Autodesk Inventor part; units mm, degrees
ref_plane "YZ Plane" through (0, 0, 0) normal (1, 0, 0) x (0, 1, 0)
ref_plane "XZ Plane" through (0, 0, 0) normal (0, 1, 0) x (-1, 0, 0)
ref_plane "XY Plane" through (0, 0, 0) normal (0, 0, 1) x (1, 0, 0)
sketch "Boceto1" plane through (0, 0, 0) normal (0, 1, 0) x (-1, 0, 0)
  circle A0 centre (-59.7419, -103.4763) radius 7.9656
  circle A1 centre (-47.2958, -81.9187) radius 1.9914
  line L0 (-73.6817, -103.4763) -> (-73.6817, 5.1739)
  line L1 (32.3603, -66.3972) -> (-52.772, -115.5485)
  arc A2 (-73.6817, -103.4763) -> (-52.772, -115.5485) centre (-59.7419, -103.4763) ccw
  line L2 (13.9398, -24.1443) -> (18.9183, -32.7673)
  line L3 (20.9097, -36.2166) -> (25.8882, -44.8396)
  line L4 (27.8796, -48.2888) -> (32.8581, -56.9118)
  line L5 (7.5794, -22.7716) -> (11.1559, -28.9662)
  line L6 (11.1559, -28.9662) -> (13.9398, -24.1443)
  line L7 (13.9398, -24.1443) -> (18.9183, -32.7673)
  line L8 (18.9183, -32.7673) -> (12.9441, -32.7673)
  line L9 (12.9441, -32.7673) -> (17.9226, -41.3904)
  line L10 (17.9226, -41.3904) -> (20.9097, -36.2166)
  line L11 (20.9097, -36.2166) -> (25.8882, -44.8396)
  line L12 (25.8882, -44.8396) -> (19.914, -44.8396)
  line L13 (19.914, -44.8396) -> (24.8925, -53.4626)
  line L14 (24.8925, -53.4626) -> (27.8796, -48.2888)
  line L15 (27.8796, -48.2888) -> (32.8581, -56.9118)
  line L16 (32.8581, -56.9118) -> (26.8839, -56.9118)
  line L17 (26.8839, -56.9118) -> (32.3603, -66.3972)
  line L18 (-27.8795, 0.0001) -> (-37.8365, 0.0001)
  line L19 (-41.8193, 0.0001) -> (-51.7763, 0.0001)
  line L20 (-55.7591, 0.0001) -> (-65.7161, 0.0001)
  line L21 (-23.4355, 5.1739) -> (-30.8666, 5.1739)
  line L22 (-30.8666, 5.1739) -> (-27.8795, 0.0001)
  line L23 (-27.8795, 0.0001) -> (-37.8365, 0.0001)
  line L24 (-37.8365, 0.0001) -> (-34.8494, 5.1739)
  line L25 (-34.8494, 5.1739) -> (-44.8064, 5.1739)
  line L26 (-44.8064, 5.1739) -> (-41.8193, 0.0001)
  line L27 (-41.8193, 0.0001) -> (-51.7763, 0.0001)
  line L28 (-51.7763, 0.0001) -> (-48.7892, 5.1739)
  line L29 (-48.7892, 5.1739) -> (-58.7462, 5.1739)
  line L30 (-58.7462, 5.1739) -> (-55.7591, 0.0001)
  line L31 (-55.7591, 0.0001) -> (-65.7161, 0.0001)
  line L32 (-65.7161, 0.0001) -> (-62.729, 5.1739)
  line L33 (-62.729, 5.1739) -> (-73.6817, 5.1739)
  arc A3 (-23.4355, 5.1739) -> (7.5794, -22.7716) centre (0, 0) ccw
extrude "Extrusión2" add sketch "Boceto1" along normal blind 10
sketch "Boceto2" plane through (0, 10, 0) normal (0, 1, 0) x (1, 0, 0)
  circle A0 centre (59.7419, 103.4763) radius 7.9656
  circle A1 centre (47.2958, 81.9187) radius 1.9914
  arc A2 (73.6817, 103.4763) -> (52.772, 115.5485) centre (59.7419, 103.4763) ccw
  line L0 (52.772, 115.5485) -> (-32.3603, 66.3972)
  line L1 (-32.3603, 66.3972) -> (-26.8839, 56.9118)
  line L2 (-26.8839, 56.9118) -> (-32.8581, 56.9118)
  line L3 (-32.8581, 56.9118) -> (-27.8796, 48.2888)
  line L4 (-27.8796, 48.2888) -> (-24.8925, 53.4626)
  line L5 (-24.8925, 53.4626) -> (-19.914, 44.8396)
  line L6 (-19.914, 44.8396) -> (-25.8882, 44.8396)
  line L7 (-25.8882, 44.8396) -> (-20.9097, 36.2166)
  line L8 (-20.9097, 36.2166) -> (-17.9226, 41.3904)
  line L9 (-17.9226, 41.3904) -> (-12.9441, 32.7673)
  line L10 (-12.9441, 32.7673) -> (-18.9183, 32.7673)
  line L11 (-18.9183, 32.7673) -> (-13.9398, 24.1443)
  line L12 (-13.9398, 24.1443) -> (-11.1559, 28.9662)
  line L13 (-11.1559, 28.9662) -> (-7.5794, 22.7716)
  arc A3 (23.4355, -5.1739) -> (-7.5794, 22.7716) centre (0, 0) ccw
  line L14 (23.4355, -5.1739) -> (30.8666, -5.1739)
  line L15 (30.8666, -5.1739) -> (27.8795, -0.0001)
  line L16 (27.8795, -0.0001) -> (37.8365, -0.0001)
  line L17 (37.8365, -0.0001) -> (34.8494, -5.1739)
  line L18 (34.8494, -5.1739) -> (44.8064, -5.1739)
  line L19 (44.8064, -5.1739) -> (41.8193, -0.0001)
  line L20 (41.8193, -0.0001) -> (51.7763, -0.0001)
  line L21 (51.7763, -0.0001) -> (48.7892, -5.1739)
  line L22 (48.7892, -5.1739) -> (58.7462, -5.1739)
  line L23 (58.7462, -5.1739) -> (55.7591, -0.0001)
  line L24 (55.7591, -0.0001) -> (65.7161, -0.0001)
  line L25 (65.7161, -0.0001) -> (62.729, -5.1739)
  line L26 (62.729, -5.1739) -> (73.6817, -5.1739)
  line L27 (73.6817, -5.1739) -> (73.6817, 103.4763)
  line L28 (-2.0722, 33.9367) -> (-18.7001, 62.7369)
  line L29 (-18.7001, 62.7369) -> (29.3976, 90.5062)
  circle A4 centre (47.2958, 81.9187) radius 1.9914
  line L30 (52.772, 115.5485) -> (-32.3603, 66.3972)
  arc A5 (12.4849, 31.6246) -> (-2.0722, 33.9367) centre (0, 0) ccw
  circle A6 centre (59.7419, 103.4763) radius 7.9656
  arc A7 (29.3976, 90.5062) -> (39.1023, 77.7274) centre (59.7419, 103.4763) ccw
  line L31 (12.4849, 31.6246) -> (39.1023, 77.7274)
  line L32 (0, 0) -> (59.7419, 103.4763)
  line L33 (32.4961, 9.9999) -> (63.6817, 9.9999)
  line L34 (63.6817, 9.9999) -> (63.6817, 70.7123)
  line L35 (21.1452, 26.6246) -> (47.7626, 72.7274)
  arc A8 (47.7626, 72.7274) -> (63.6817, 70.7123) centre (59.7419, 103.4763) ccw
  arc A9 (32.4961, 9.9999) -> (21.1452, 26.6246) centre (0, 0) ccw
  line L36 (41.8193, -0.0001) -> (51.7763, -0.0001)
  line L37 (73.6817, -5.1739) -> (73.6817, 103.4763)
  dimension "d6" = 10
  dimension "d8" = 10
  dimension "d10" = 33
  dimension "d11" = 5
  dimension "d12" = 10
  dimension "d13" = 10
  dimension "d14" = 10
  dimension "d15" = 10
  dimension "d16" = 33
  dimension "d17" = 5
The listing builds one solid part. Answer for the finished solid, in the listing's coordinates (mm). A direction names the side the tool comes from. Coordinates: 2 decimals unless noted, no trailing zeros. Loops run counter-clockwise (first coordinate to the right, second up) from the corner with the lowest first, then second, coordinate; pieces in that order, holes last.
1) Find section D-D on x = 5.5. Write down the section's boundary in (y, z), then the cut area to 3 significant figures.
2) A tool of negligible diameter and unlimited length cuts with its end or side. For faces 4 (the face through (43.33, 4.93, 2.62)), 5 (the face through (66.53, 4.93, -115.65)), from which of +Z, -Z, +X, -X, +Y, -Y can it reach the whole face along a straight path? Write none if from no direction.
3) Determine the mould class of faces 1 (the face through (47, 5, 0)), 2 (the face through (73.682, 5, -50)), 3 (the face through (-30.334, 4.93, -52.54)) for opening direction X: pulls with the +X half, pulls with the -X half, needs draft (parallel to the pull), parting line crosses it, or undercut.
4) Find section B-B on x = -22.5. Write down the section's boundary in (y, z).
5) Find the intervals of material crossed by L1, parallel to X at y = 4, z = -1; L2, parallel to X at y = 5.75, z = -26; L3, parallel to Z at x = 35.5, y = 6.75, in increasing order.
6) Find section A-A on z = -97. Write down the section's boundary in (x, y), then the cut area to 3 significant figures.
7) Flat-ended cylindrical pins translate along their axes: pin 1 Ø5 at (x, y) = (39, 8) entering from -Z; pin 2 Ø3 at (y, z) = (5.5, -32.5) entering from -X; pin 3 Ø5 at (y, z) = (7, -7.5) entering from -X. Find the tip coordinate at first contact, or state that the pin passes through.
8) Find section C-C on y = 5. Give the number of separate pieces and of enclosed holes in the cut face, then the cut area to 3 significant figures.
Values:
1. outline: (0, -88.26) - (10, -88.26) - (10, -23.36) - (0, -23.36) - close
1. area: 649 mm2
2. face 4: +Y, -Y
2. face 5: -Z, +Y, -Y
3. face 1: undercut
3. face 2: pulls with the +X half
3. face 3: pulls with the -X half
4. outline: (0, -72.09) - (10, -72.09) - (10, -49.32) - (0, -49.32) - close; (0, -44.84) - (10, -44.84) - (10, -38.97) - (0, -38.97) - close
5. L1: x = 23.98 to 73.68
5. L2: x = -15.01 to -12.87, -9.44 to 73.68
5. L3: z = -105.58 to 0, 4.05 to 5.17
6. outline: (20.65, 0) - (55.1, 0) - (55.1, 10) - (20.65, 10) - close; (64.38, 0) - (73.68, 0) - (73.68, 10) - (64.38, 10) - close
6. area: 438 mm2
7. pin 1: stops at z = -109.04
7. pin 2: stops at x = -18.92
7. pin 3: stops at x = 21.82
8. separate pieces: 1
8. enclosed holes: 2
8. area: 8,460 mm2
